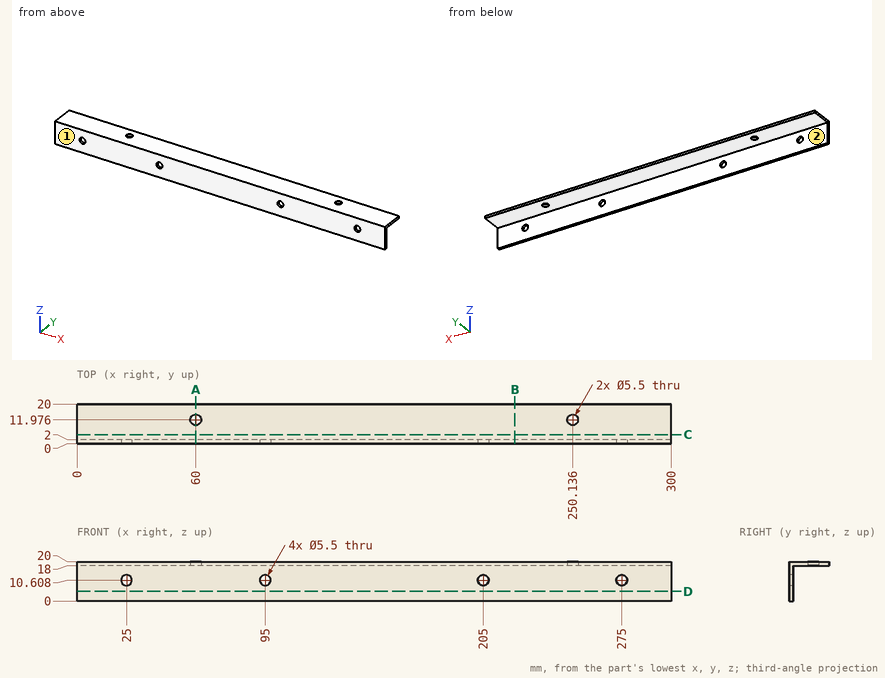
The drawing under review shows one solid part. Ordinate dimensions are in mm from its lowest x, y, z. A direction names the side the tool comes from. Coordinates: 2 decimals unless noted, no trailing zeros. Write each loop counter-clockwise with the first axis right and the second up, starting at its lowest first coordinate (ties: lowest second). Pieces come first, ordered by that corner, then holes. Notation, with made-up numbers: (77, -33) -> (88, -33) arc R26 ccw to (88, -17) -> close; hole circle Ø2 at (75, 88.5). An arc over 180 degrees is marked (long way). Write each question's results on one line, items separated by ' | '. Start each with the question number.
1) Wall thickness on L1, parallel to Z at x = 205, y = 1.3; L2, parallel to Y at x = 60, z = 19.2 (1 decimal); L3, parallel to Z at x = 141.5, y = 12.5: over which ranges is each line inside the solid? List them lowest first. Write a range as [from, to].
2) Consider section B-B (x = 221). Write out the cut boundary in (y, z).
3) For the marked faces 1 and 2, list the 3-axis set-ups (+Z, -Z, +X, -X, +Y, -Y) from which the entire face can be reached by the end or side of a thin tool; tool diameter is ignored.
4) Insertion check: pin 1 (5 mm diameter, centred on x = 60, y = 11.98, fed in from +Z); pin 2 (4 mm diameter, centred on x = 124, y = 5.5, fed in from -Z); pin 3 (6.5 mm diameter, centred on x = 25, z = 10.61, fed in from +Y). Each pin has a flat end and moves straight along its axis. Give the tip position at first contact, or say it passes through.
5) Consider section C-C (y = 4.5). Write out the cut boundary in (x, z).
6) Consider section D-D (z = 5). Write out the cut boundary in (x, y).
7) Consider section A-A (x = 60). Write out the cut boundary in (y, z) (1 decimal).
Geometry says:
1) L1: [0, 7.86], [13.36, 20] | L2: [0, 9.2], [14.7, 20] | L3: [18, 20]
2) outline: (0, 0) -> (2, 0) -> (2, 18) -> (20, 18) -> (20, 20) -> (0, 20) -> close
3) face 1: +Z, -Z, +X, -X, -Y | face 2: -Z, +X, -X, +Y
4) pin 1: through | pin 2: z = 18 | pin 3: y = 2
5) outline: (0, 18) -> (300, 18) -> (300, 20) -> (0, 20) -> close
6) outline: (0, 0) -> (300, 0) -> (300, 2) -> (0, 2) -> close
7) outline: (0, 0) -> (2, 0) -> (2, 18) -> (9.2, 18) -> (9.2, 20) -> (0, 20) -> close; (14.7, 18) -> (20, 18) -> (20, 20) -> (14.7, 20) -> close
